Geometry check sheet. Reference: the model listing, model coordinates, mm. Face numbers are marked on the shaded views. A direction names the side the tool comes from. Give positions to 0.01 mm unless a question says otherwise; leave off trailing zeros. Loops run counter-clockwise (first coordinate to the right, second up) from the corner with the lowest first, then second, coordinate; pieces in that order, holes last. Notation, with made-up numbers: (30, 71.5) -> (48, 71.5) arc R19 cw to (48, 82.5) -> close; hole circle Ø1 at (44, 69). An arc over 180 degrees is marked (long way). One line per item, written item: value. Start each with the question number.
(1) Sectioned sample at C-C, the plane x = 0. Record the cut outline in (y, z), then the cut area to 3 significant figures.
(2) Scan lines: line 1 along X through (y, z) = (-36, 8.25); line 2 along X through (y, z) = (0, 5); line 3 along Y through (x, z) = (-14, 6.5). Record each from-to range of solid material in increasing order. Write a range as from..to.
(3) Tool access check on the marked faces 5, 6 and 7. Record the directions out of +Z, -Z, +X, -X, +Y, -Y that give a thin tool (end or side, any length) a straight path to the whole face; none if there is none.
(4) Gauge pin test, flat ends, axial feed: pin 1 Ø1.5 at (y, z) = (-18.5, 13.5) entering from +X; pin 2 Ø12 at (x, y) = (-11.5, 6) entering from +Z; pin 3 Ø4 at (x, z) = (4.5, 11.5) entering from +Y. Record the tip position at first contact, or that the pin passes through.
(5) Sectioned sample at D-D, the plane y = 18. Record the cut outline in (x, z).
(6) Sectioned sample at B-B, the plane z = 6. Record the cut outline in (x, y), then the cut area to 3 significant figures.
(7) Sectioned sample at A-A, the plane y = 0. Record the cut outline in (x, z).
(8) Draft check along X on the marked faces 1, 2, 3 and 4. Enter one of: pulls with the +X half, pulls with the -X half, needs draft (parallel to the pull), parting line crosses it, or undercut.
from build123d import *

# Parameters (mm, degrees)
F0_R     = 25
F1_DEPTH = 15.86
F2_R     = 23
F3_DEPTH = 13.7
F4_W     = 21
F4_H     = 21
F5_DEPTH = 15.86
F6_W     = 17
F6_H     = 21
F7_DEPTH = 13.7


with BuildPart() as f1:
    # F0 (on Top) → F1 (new body)
    with BuildSketch(Plane.XY):
        Circle(F0_R)
    extrude(amount=F1_DEPTH)

    # F2 (on face) → F3 (cut)
    with BuildSketch(Plane.XY.offset(15.86)):
        Circle(F2_R)
    extrude(amount=-F3_DEPTH, mode=Mode.SUBTRACT)

    # F4 (on Top) → F5 (join, through all)
    with BuildSketch(Plane.XY):
        with Locations((0, -30.9633819297)):
            Rectangle(F4_W, F4_H)
    extrude(amount=F5_DEPTH)

    # F6 (on face) → F7 (cut, through all)
    with BuildSketch(Plane.XY.offset(15.86)):
        with Locations((0, -30.9633819297)):
            Rectangle(F6_W, F6_H)
    extrude(amount=-F7_DEPTH, mode=Mode.SUBTRACT)


solid = f1.part
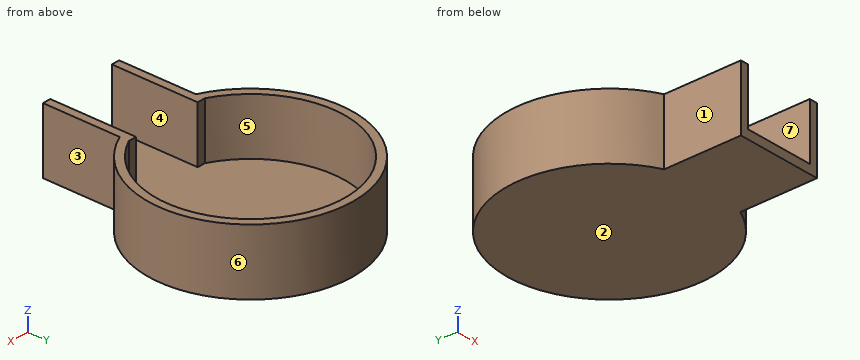
Calculated:
1. outline: (-41.46, 0) -> (25, 0) -> (25, 15.86) -> (23, 15.86) -> (23, 2.16) -> (-41.46, 2.16) -> close
1. area: 171 mm2
2. line 1: x = -10.5..-8.5, 8.5..10.5
2. line 2: x = -25..-23, 23..25
2. line 3: y = -20.71..-18.25, 18.25..20.71
3. face 5: +Z
3. face 6: +Z, -Z
3. face 7: +Z, -Y
4. pin 1: stops at x = 17.61
4. pin 2: stops at z = 2.16
4. pin 3: stops at y = 24.87
5. outline: (-17.35, 0) -> (17.35, 0) -> (17.35, 15.86) -> (14.32, 15.86) -> (14.32, 2.16) -> (-14.32, 2.16) -> (-14.32, 15.86) -> (-17.35, 15.86) -> close
6. outline: (-10.5, -41.46) -> (-8.5, -41.46) -> (-8.5, -20.46) -> (-10.5, -20.46) arc R23 cw (long way) to (10.5, -20.46) -> (8.5, -20.46) -> (8.5, -41.46) -> (10.5, -41.46) -> (10.5, -22.69) arc R25 ccw (long way) to (-10.5, -22.69) -> close
6. area: 342 mm2
7. outline: (-25, 0) -> (25, 0) -> (25, 15.86) -> (23, 15.86) -> (23, 2.16) -> (-23, 2.16) -> (-23, 15.86) -> (-25, 15.86) -> close
8. face 1: pulls with the -X half
8. face 2: needs draft
8. face 3: pulls with the +X half
8. face 4: undercut
